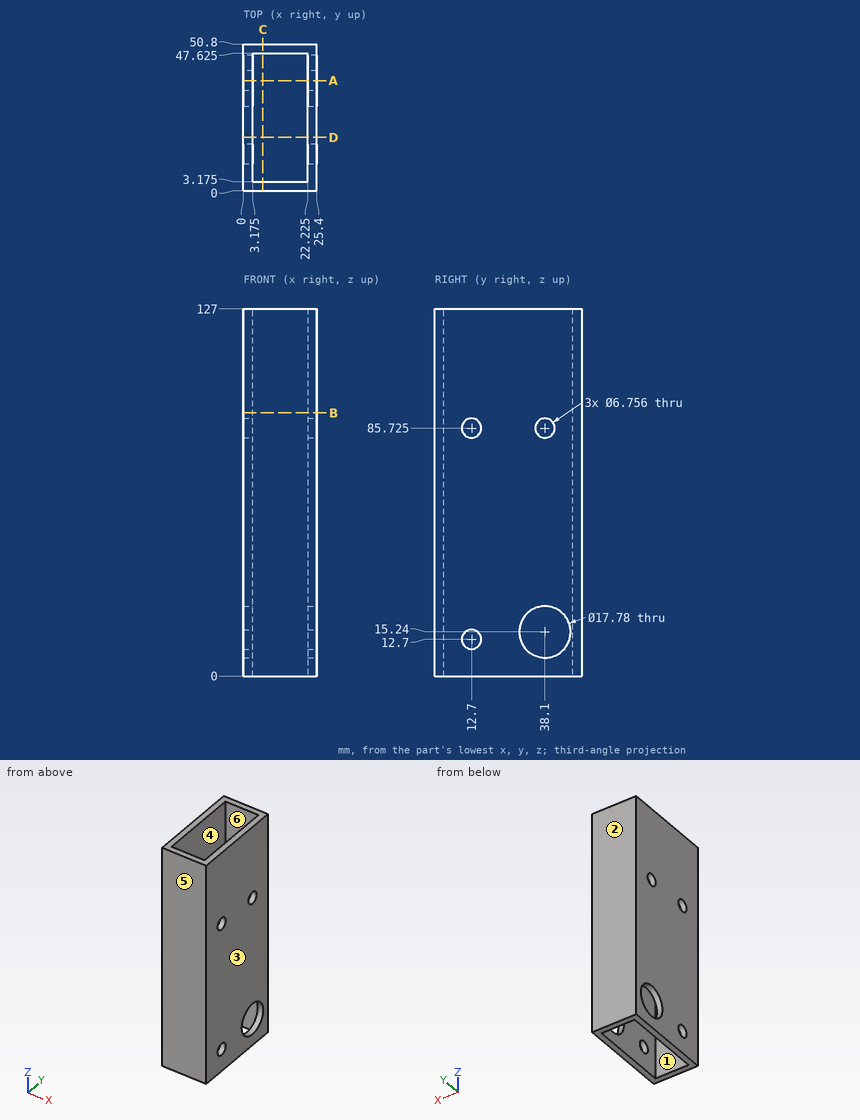
Part print with two shaded views. Sizes in mm from the minimum x, y, z corner. A direction names the side the tool comes from. Coordinates: 2 decimals unless noted, no trailing zeros. Write each loop counter-clockwise with the first axis right and the second up, starting at its lowest first coordinate (ties: lowest second). Pieces come first, ordered by that corner, then holes.
1. Band-saw the part on C-C, the plane x = 6.75. Give the cut face in (y, z) (1 decimal).
Answer block:
outline: (0, 0) - (3.2, 0) - (3.2, 127) - (0, 127) - close; (47.6, 0) - (50.8, 0) - (50.8, 127) - (47.6, 127) - close
2. Band-saw the part on B-B, the plane z = 91. Give the cut face in (x, y) (1 decimal).
Answer block:
outline: (0, 0) - (25.4, 0) - (25.4, 50.8) - (0, 50.8) - close; hole (3.2, 3.2) - (22.2, 3.2) - (22.2, 47.6) - (3.2, 47.6) - close
3. Drill centre lines: probe 1 along Z at (x, y) = (24.1, 12.7); probe 2 along Z at (x, y) = (23.6, 38.1); probe 3 along X at (y, z) = (5.5, 108) (1 decimal). Where is each one in solid material? Low to high.
Answer block:
probe 1: z = 0 to 9.32, 16.08 to 82.35, 89.1 to 127
probe 2: z = 0 to 6.35, 24.13 to 82.35, 89.1 to 127
probe 3: x = 0 to 3.2, 22.2 to 25.4
4. Band-saw the part on D-D, the plane y = 18.5. Give the cut face in (x, z) (1 decimal).
Answer block:
outline: (0, 0) - (3.2, 0) - (3.2, 127) - (0, 127) - close; (22.2, 0) - (25.4, 0) - (25.4, 127) - (22.2, 127) - close
5. 3-axis set-ups, long thin cutter, end or side, ignore diameter. For the marked faces 5 and 6: which of +Z, -Z, +X, -X, +Y, -Y reach the whole face in a straight line?
Answer block:
face 5: +Z, -Z, +X, -X, -Y
face 6: +Z, -Z
6. Pull direction X, two halves, no side cores. Call the marked faces 1, 2, 3 and 4: released by +X, released by -X, zero draft, split by the parting line, or undercut.
Answer block:
face 1: undercut
face 2: zero draft
face 3: released by +X
face 4: undercut
7. Drop flat-ended pins along their axis: pin 1 (8 mm diameter, centred on x = 21.5, y = 44, fed in from +Z); pin 2 (10.5 mm diameter, centred on y = 38.1, z = 15.24, fed in from +X). Give the stop position or say it passes through.
Answer block:
pin 1: stops at z = 127
pin 2: passes through
8. Band-saw the part on A-A, the plane y = 38.1. Give the number of separate pieces and of enclosed holes in the cut face.
Answer block:
separate pieces: 6
enclosed holes: 0
